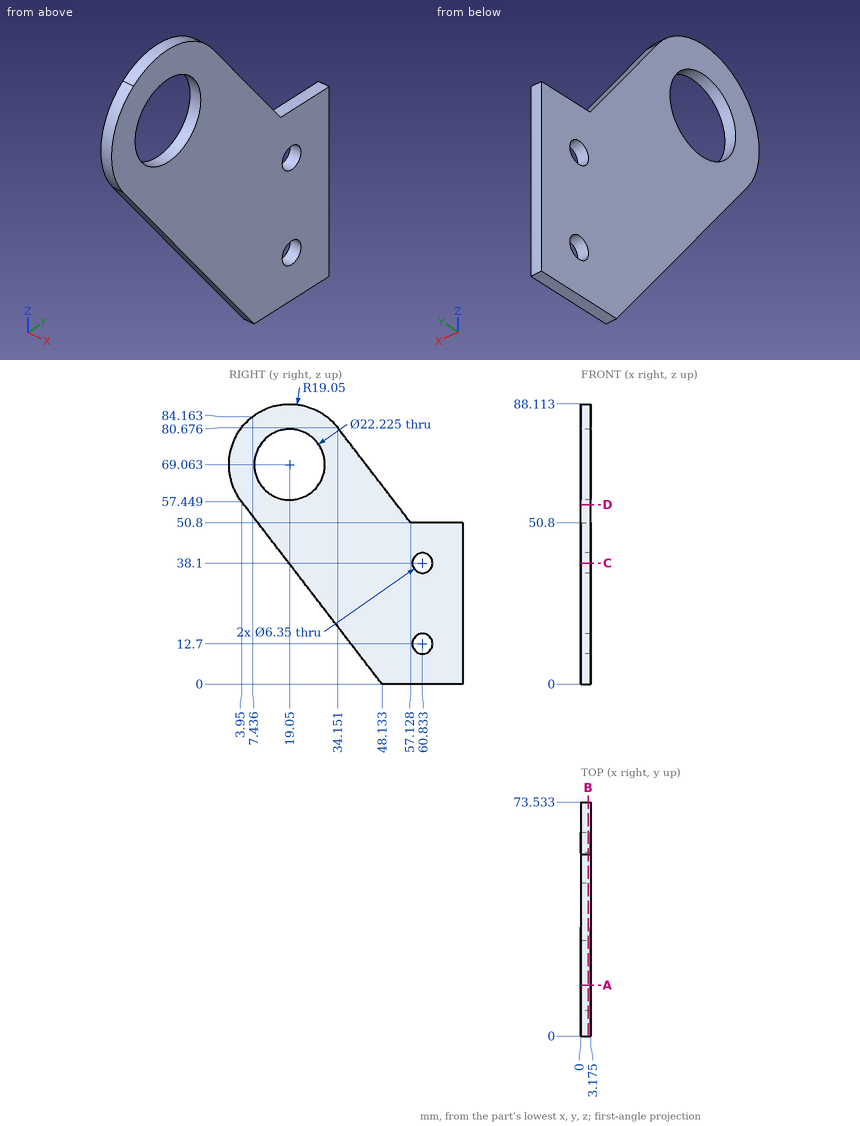
Could you check a few things on this drawing? It's one solid part, dimensions in mm from its lowest x, y, z. Coordinates: 2 decimals unless noted, no trailing zeros. Order: outer loops, then holes, each group sorted by start corner. A loop starts at its lowest first (then second) coordinate and runs counter-clockwise, first axis right, second up.
1. If we section it at C-C (z = 38.1): Please give me the cut outline in (x, y) (1 decimal).
2. I need wall thicknesses on line 1 (Z direction, x = 2, y = 10.5) (1 decimal); line 2 (Z direction, x = 0.4, y = 18) (1 decimal); line 3 (Z direction, x = 1.8, y = 68). Which ranges of each line are inside material? Lowest first, please.
3. If we section it at B-B (x = 2.3): Give the number of separate pieces and of enclosed holes in the cut face, then the cut area to 3 significant figures.
4. If we section it at A-A (y = 16): Please give me the cut outline in (x, z) (1 decimal).
5. I'm going to push flat-ended pins straight in: pin 1 (1.5 mm diameter, centred on x = 1.5, y = 44, fed in from -Z); pin 2 (4 mm diameter, centred on y = 60.83, z = 38.1, fed in from -X); pin 3 (8.5 mm diameter, centred on y = 60.83, z = 12.7, fed in from +X) (1 decimal); pin 4 (1.6 mm diameter, centred on x = 1.5, y = 67, fed in from +Z). Where does each tip first touch, or does it pass through?
6. If we section it at D-D (z = 56.5): Please give me the cut outline in (x, y) (1 decimal), then the cut area to 3 significant figures.
Entries:
1. outline: (0, 18.8) - (3.2, 18.8) - (3.2, 57.7) - (0, 57.7) - close; (0, 64) - (3.2, 64) - (3.2, 73.5) - (0, 73.5) - close
2. line 1: z = 48.9 to 62, 76.2 to 86.1
2. line 2: z = 39.2 to 58, 80.1 to 88.1
2. line 3: z = 0 to 50.8
3. separate pieces: 1
3. enclosed holes: 3
3. area: 3,280 mm2
4. outline: (0, 41.8) - (3.2, 41.8) - (3.2, 58.4) - (0, 58.4) - close; (0, 79.7) - (3.2, 79.7) - (3.2, 87.9) - (0, 87.9) - close
5. pin 1: stops at z = 4.4
5. pin 2: passes through
5. pin 3: stops at x = 3.2
5. pin 4: stops at z = 50.8
6. outline: (0, 4.7) - (3.2, 4.7) - (3.2, 52.7) - (0, 52.7) - close
6. area: 153 mm2
